```python
from build123d import *

# Parameters (mm, degrees)
SKETCH1_W           = 25
SKETCH1_H           = 25
BOSS_EXTRUDE1_DEPTH = 10
FILLET1_R           = 3
SKETCH2_R           = 1.3
CUT_EXTRUDE1_DEPTH  = 10
SKETCH3_R           = 11.95
CUT_EXTRUDE2_DEPTH  = 10


with BuildPart() as part:
    # Sketch1 → Boss-Extrude1 (new body)
    with BuildSketch(Plane.XY):
        with Locations((-25.324193791, -75.114139951)):
            Rectangle(SKETCH1_W, SKETCH1_H)
    extrude(amount=BOSS_EXTRUDE1_DEPTH)

    # Fillet1
    fillet1_edges = [part.edges().sort_by_distance(p)[0] for p in [
        (-12.824193791, -87.614139951, 5),
        (-37.824193791, -87.614139951, 5),
        (-37.824193791, -62.614139951, 5),
        (-12.824193791, -62.614139951, 5),
    ]]
    fillet(fillet1_edges, radius=FILLET1_R)

    # Sketch2 → Cut-Extrude1 (cut)
    with BuildSketch(Plane.XY.offset(10)):
        with Locations((-15.324193791, -85.114139951)):
            Circle(SKETCH2_R)
        with Locations((-15.324193791, -65.114139951)):
            Circle(SKETCH2_R)
        with Locations((-35.324193791, -65.114139951)):
            Circle(SKETCH2_R)
        with Locations((-35.324193791, -85.114139951)):
            Circle(SKETCH2_R)
    extrude(amount=-CUT_EXTRUDE1_DEPTH, mode=Mode.SUBTRACT)

    # Sketch3 → Cut-Extrude2 (cut)
    with BuildSketch(Plane.XY.offset(10)):
        with Locations((-25.324193791, -75.114139951)):
            Circle(SKETCH3_R)
    extrude(amount=-CUT_EXTRUDE2_DEPTH, mode=Mode.SUBTRACT)


solid = part.part
```
Model file for the job. Use its own axes, mm. Coordinates: 2 decimals unless noted, no trailing zeros. Loops run counter-clockwise (first coordinate to the right, second up) from the corner with the lowest first, then second, coordinate; pieces in that order, holes last. Notation, with made-up numbers: (50.25, 14.25) - (84.25, 14.25) arc R25 ccw to (84.25, 40.25) - close; hole circle Ø5 at (-30.75, 14.25). An arc over 180 degrees is marked (long way). Write item = value, one per line. Start each with the question number.
Item 1: Pull direction X, two halves, no side cores. Call faces 1 (the face through (-36.97, -63.52, 5.07)), 2 (the face through (-25, -62.614, 5)), 3 (the face through (-18.9, -65.04, 5.07)): +X half, -X half, draft (parallel to the pull), parting line (faces both ways), or undercut.
Item 2: Wall check: probe 1 along X at (y, z) = (-75, 5.75); probe 2 along X at (y, z) = (-66.25, 4.5); probe 3 along Y at (x, z) = (-16, 1.25). Give the ranges that are in metal, low to high. Write a range as [from, to].
Item 3: Saw through at C-C, the plane z = 4.5. List the corners of the cut face in (x, y).
Item 4: Drop a flat-ended pin along its axis: pin 1 Ø2 at (x, y) = (-35.32, -85.11) entering from -Z. Give the stop position or say it passes through.
Item 5: Saw through at A-A, the plane y = -72.5. List the corners of the cut face in (x, z), then the cut area to 3 significant figures.
Item 6: Saw through at D-D, the plane y = -86. List the corners of the cut face in (x, z), then the cut area to 3 significant figures.
Item 7: Saw through at B-B, the plane x = -33. List the corners of the cut face in (y, z), then the cut area to 3 significant figures.
Answers:
q1.face_1 = -X half
q1.face_2 = draft
q1.face_3 = undercut
q2.probe_1 = [-37.82, -37.27], [-13.37, -12.82]
q2.probe_2 = [-37.82, -35.96], [-34.69, -33.34], [-17.31, -15.96], [-14.69, -12.82]
q2.probe_3 = [-87.61, -86.22], [-84, -82.59], [-67.64, -66.22], [-64, -62.61]
q3.outline = (-37.82, -84.61) arc R3 ccw to (-34.82, -87.61) - (-15.82, -87.61) arc R3 ccw to (-12.82, -84.61) - (-12.82, -65.61) arc R3 ccw to (-15.82, -62.61) - (-34.82, -62.61) arc R3 ccw to (-37.82, -65.61) - close; hole circle Ø23.9 at (-25.32, -75.11); hole circle Ø2.6 at (-35.32, -85.11); hole circle Ø2.6 at (-35.32, -65.11); hole circle Ø2.6 at (-15.32, -85.11); hole circle Ø2.6 at (-15.32, -65.11)
q4.pin_1 = through
q5.outline = (-37.82, 0) - (-36.98, 0) - (-36.98, 10) - (-37.82, 10) - close; (-13.66, 0) - (-12.82, 0) - (-12.82, 10) - (-13.66, 10) - close
q5.area = 16.8 mm2
q6.outline = (-37.48, 0) - (-36.28, 0) - (-36.28, 10) - (-37.48, 10) - close; (-34.37, 0) - (-30.25, 0) - (-30.25, 10) - (-34.37, 10) - close; (-20.39, 0) - (-16.28, 0) - (-16.28, 10) - (-20.39, 10) - close; (-14.37, 0) - (-13.16, 0) - (-13.16, 10) - (-14.37, 10) - close
q6.area = 107 mm2
q7.outline = (-87.61, 0) - (-84.27, 0) - (-84.27, 10) - (-87.61, 10) - close; (-65.96, 0) - (-62.61, 0) - (-62.61, 10) - (-65.96, 10) - close
q7.area = 66.8 mm2
